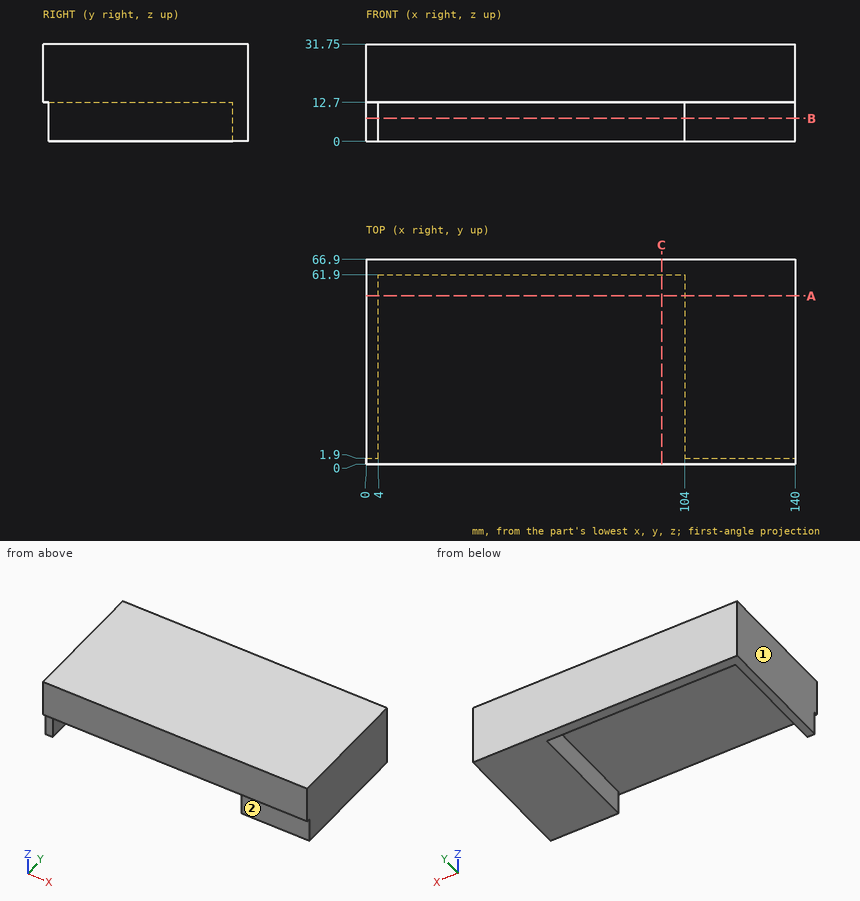
Geometry check sheet. Reference: drawing and pictorial views, mm from the part's lowest x, y, z. A direction names the side the tool comes from. Round coordinates to 2 decimals unless told otherwise and drop trailing zeros. Loops run counter-clockwise (first coordinate to the right, second up) from the corner with the lowest first, then second, coordinate; pieces in that order, holes last. Notation, with made-up numbers: (39.25, -22) - (73.25, -22) arc R31 ccw to (73.25, 7) - close; hole circle Ø9 at (-6.5, 72.5). An arc over 180 degrees is marked (long way). Use a Markdown table: item, result. Add a question column.
1. Section check C-C, the plane x = 96.5. Record the boundary of the cut face in (y, z).
2. Thickness scan on probe 1 along X at (y, z) = (41.5, 5); probe 2 along Z at (x, y) = (15.5, 43.5); probe 3 along Y at (x, z) = (118.5, 11). Record the ranges inside material, lowest first. Write a range as [from, to].
3. Section check B-B, the plane z = 7.5. Record the boundary of the cut face in (x, y), plus the area to 3 significant figures.
4. Gauge pin test, flat ends, axial feed: pin 1 (12 mm diameter, centred on x = 24, y = 25.5, fed in from -Z); pin 2 (12 mm diameter, centred on x = 101, y = 26, fed in from -Z); pin 3 (2 mm diameter, centred on x = 2.5, z = 6, fed in from -Y); pin 4 (6.5 mm diameter, centred on x = 42, z = 4, fed in from -Y). Record the tip position at first contact, or that the pin passes through.
5. Access from +Z, -Z, +X, -X, +Y, -Y to the whole of each face (thin tool, end or side, straight path). Record for the marked faces 1 and 2.
6. Section check A-A, the plane y = 55. Record the boundary of the cut face in (x, z).
Checks:
| question | item | result |
|---|---|---|
| 1 | outline | (0, 12.7) - (61.9, 12.7) - (61.9, 0) - (66.9, 0) - (66.9, 31.75) - (0, 31.75) - close |
| 2 | probe 1 | x = [0, 4], [104, 140] |
| 2 | probe 2 | z = [12.7, 31.75] |
| 2 | probe 3 | y = [1.9, 66.9] |
| 3 | outline | (0, 1.9) - (4, 1.9) - (4, 61.9) - (104, 61.9) - (104, 1.9) - (140, 1.9) - (140, 66.9) - (0, 66.9) - close |
| 3 | area | 3,100 mm^2 |
| 4 | pin 1 | stops at z = 12.7 |
| 4 | pin 2 | stops at z = 0 |
| 4 | pin 3 | stops at y = 1.9 |
| 4 | pin 4 | stops at y = 61.9 |
| 5 | face 1 | +Z, -Z, -X, +Y, -Y |
| 5 | face 2 | -Z, +X, -X, -Y |
| 6 | outline | (0, 0) - (4, 0) - (4, 12.7) - (104, 12.7) - (104, 0) - (140, 0) - (140, 31.75) - (0, 31.75) - close |
